The listing builds one solid part. Answer for the finished solid, in the listing's coordinates (mm). A direction names the side the tool comes from. Give positions to 0.01 mm unless a question says otherwise; leave off trailing zeros. Order: outer loops, then holes, each group sorted by start corner. A loop starts at its lowest first (then second) coordinate and runs counter-clockwise, first axis right, second up. Notation, with made-up numbers: (74.5, 83.5) -> (104.5, 83.5) arc R15 ccw to (104.5, 98.5) -> close; hole circle Ø7 at (18.5, 49.25). An arc over 180 degrees is marked (long way). One line per question, with ' | ' between items. Start each with the question number.
```python
from build123d import *

# Parameters (mm, degrees)
F1_DEPTH      = 208
F2_R          = 6
F3_DEPTH      = 65.001
F3_DEPTH_BACK = 5.001
F5_DEPTH      = 70
F6_R          = 6
F7_DEPTH      = 70.001
F8_R          = 4.05
F8_R_2        = 5
F9_DEPTH      = 40.001


with BuildPart() as f1:
    # F0 (on Front) → F1 (new body)
    with BuildSketch(Plane.XZ):
        with BuildLine():
            ThreePointArc((0, 30), (1.4644660941, 33.5355339059), (5, 35))
            Line((5, 35), (55, 35))
            ThreePointArc((55, 35), (58.5355339059, 33.5355339059), (60, 30))
            Line((60, 30), (60, 0))
            Line((60, 0), (65, 0))
            Line((65, 0), (65, 30))
            ThreePointArc((65, 30), (62.0710678119, 37.0710678119), (55, 40))
            Line((55, 40), (5, 40))
            ThreePointArc((5, 40), (-2.0710678119, 37.0710678119), (-5, 30))
            Line((-5, 30), (-5, 0))
            Line((-5, 0), (0, 0))
            Line((0, 0), (0, 30))
        make_face()
    extrude(amount=F1_DEPTH)

    # F2 (on Right) → F3 (cut, two sides)
    with BuildSketch(Plane.YZ) as f3_sk:
        with Locations((-196.0943733454, 12)):
            Circle(F2_R)
        with Locations((-156.0943733454, 12)):
            Circle(F2_R)
        with BuildLine():
            ThreePointArc((-34.0443733454, 12), (-38.0943733454, 16.05), (-42.1443733454, 12))
            ThreePointArc((-42.1443733454, 12), (-38.0943733454, 7.95), (-34.0443733454, 12))
        make_face()
        with BuildLine():
            ThreePointArc((-92.0443733454, 12), (-96.0943733454, 16.05), (-100.1443733454, 12))
            Line((-100.1443733454, 12), (-96.0943733454, 12))
            Line((-96.0943733454, 12), (-92.0443733454, 12))
        make_face()
        with BuildLine():
            Line((-96.0943733454, 12), (-100.1443733454, 12))
            ThreePointArc((-100.1443733454, 12), (-96.0943733454, 7.95), (-92.0443733454, 12))
            Line((-92.0443733454, 12), (-96.0943733454, 12))
        make_face()
    extrude(amount=F3_DEPTH, mode=Mode.SUBTRACT)
    extrude(f3_sk.sketch, amount=-F3_DEPTH_BACK, mode=Mode.SUBTRACT)

    # F4 (on Front) → F5 (join)
    with BuildSketch(Plane.XZ):
        Polygon((-5, 0), (0, 0), (0, 54), (0, 64), (-5, 64), (-5, 54), align=None)
        Polygon((60, 64), (60, 54), (60, 0), (65, 0), (65, 54), (65, 64), align=None)
    extrude(amount=-F5_DEPTH)

    # F6 (on face) → F7 (cut, through all)
    with BuildSketch(Plane(origin=(-5, 0, 0), x_dir=(0, -1, 0), z_dir=(-1, 0, 0))):
        with Locations((-60, 54)):
            Circle(F6_R)
        with Locations((-15.6066017178, 53.3933982822)):
            Circle(F6_R)
        with Locations((-60, 10)):
            Circle(F6_R)
        with Locations((-15.6066017178, 10.6066017178)):
            Circle(F6_R)
        with BuildLine():
            Line((-70, 10), (-70, 0))
            Line((-70, 0), (-60, 0))
            ThreePointArc((-60, 0), (-67.0710678119, 2.9289321881), (-70, 10))
        make_face()
        with BuildLine():
            ThreePointArc((208, 10), (205.0710678119, 2.9289321881), (198, 0))
            Line((198, 0), (208, 0))
            Line((208, 0), (208, 10))
        make_face()
        with BuildLine():
            Line((-70, 64), (-70, 54))
            ThreePointArc((-70, 54), (-67.0710678119, 61.0710678119), (-60, 64))
            Line((-60, 64), (-70, 64))
        make_face()
        with BuildLine():
            Line((-5, 64), (-15, 64))
            ThreePointArc((-15, 64), (-7.9289321881, 61.0710678119), (-5, 54))
            Line((-5, 54), (-5, 35))
            ThreePointArc((-5, 35), (-3.5355339059, 31.4644660941), (0, 30))
            Line((0, 30), (0, 63.4983927011))
            Line((0, 63.4983927011), (0, 64))
            Line((0, 64), (-5, 64))
        make_face()
    extrude(amount=-F7_DEPTH, mode=Mode.SUBTRACT)

    # F8 (on face) → F9 (cut, through all)
    with BuildSketch(Plane.XY.offset(40)):
        with Locations((15, -7)):
            Circle(F8_R)
        with Locations((15, -39)):
            Circle(F8_R)
        with Locations((15, -97)):
            Circle(F8_R)
        with BuildLine():
            Line((24.95, -76.95), (24.95, -97))
            Line((24.95, -97), (24.95, -117.05))
            ThreePointArc((24.95, -117.05), (30, -122.1), (35.05, -117.05))
            Line((35.05, -117.05), (35.05, -76.95))
            ThreePointArc((35.05, -76.95), (30, -71.9), (24.95, -76.95))
        make_face()
        with Locations((15, -155)):
            Circle(F8_R)
        with Locations((15, -200)):
            Circle(F8_R)
        with Locations((30, -200)):
            Circle(F8_R_2)
        with BuildLine():
            Line((35.05, -59.05), (35.05, -18.95))
            ThreePointArc((35.05, -18.95), (30, -13.9), (24.95, -18.95))
            Line((24.95, -18.95), (24.95, -59.05))
            ThreePointArc((24.95, -59.05), (30, -64.1), (35.05, -59.05))
        make_face()
        with BuildLine():
            ThreePointArc((24.95, -175.05), (30, -180.1), (35.05, -175.05))
            Line((35.05, -175.05), (35.05, -134.95))
            ThreePointArc((35.05, -134.95), (30, -129.9), (24.95, -134.95))
            Line((24.95, -134.95), (24.95, -175.05))
        make_face()
        with Locations((45, -7)):
            Circle(F8_R)
        with Locations((45, -39)):
            Circle(F8_R)
        with Locations((45, -97)):
            Circle(F8_R)
        with Locations((45, -155)):
            Circle(F8_R)
        with Locations((45, -200)):
            Circle(F8_R)
    extrude(amount=-F9_DEPTH, mode=Mode.SUBTRACT)


solid = f1.part
```
(1) Determine the mould class of faces 4 (the face through (35.05, -39, 38)), 5 (the face through (62.465, 16.907, 47.536)), 6 (the face through (-5, -40, 25)) for opening direction X: pulls with the +X half, pulls with the -X half, needs draft (parallel to the pull), parting line crosses it, or undercut.
(2) For faces 1 (the face through (-2.54, 8.01, 61.15)), 2 (the face through (29.9, -64.1, 37.5)), 3 (the face through (1, -103, 33)), determine the directions among +Z, -Z, +X, -X, +Y, -Y from which every point of the face is accessible in a straight line to the end or side of a thin tool.
(3) The part is cut by section B-B on z = 26. Determine the outline of the cut face in (x, y).
(4) Consider line 1 (X direction, y = -142, z = 15); line 2 (Z direction, x = -2.5, y = 60); line 3 (Z direction, x = 49.5, y = -166.5). Determine where each line is inside the solid, lowest interval first.
(5) The part is cut by section C-C on x = 14. Determine the outline of the cut face in (y, z), plus the area to 3 significant figures.
(6) Given P1, Ø1.5, axis at y = -94.5, z = 35, coming from the -X side; P2, Ø13, axis at x = 15, y = -97, coming from the +Z side; P3, Ø5.5, axis at x = -3.5, z = 45.5, coming from the -Y side; P4, Ø6.5, axis at y = -96.09, z = 12, coming from the +X side, each flat-ended and moving along its own axis, determine where each tip first touches the part or whether it passes through.
(7) The part is cut by section A-A on y = -7. Determine the outline of the cut face in (x, z).
(8) The part is cut by section D-D on x = 28.5. Determine the outline of the cut face in (y, z), plus the area to 3 significant figures.
Result sheet:
1) face 4: undercut | face 5: needs draft | face 6: pulls with the -X half
2) face 1: +Z, +X, -X, -Y | face 2: +Z, -Z | face 3: -Z, +Y, -Y
3) outline: (-5, -208) -> (0, -208) -> (0, 70) -> (-5, 70) -> close; (60, -208) -> (65, -208) -> (65, 70) -> (60, 70) -> close
4) line 1: x = -5 to 0, 60 to 65 | line 2: z = 0 to 4, 16 to 48, 60 to 64 | line 3: z = 35 to 40
5) outline: (-208, 35) -> (-203.92, 35) -> (-203.92, 40) -> (-208, 40) -> close; (-196.08, 35) -> (-158.92, 35) -> (-158.92, 40) -> (-196.08, 40) -> close; (-151.08, 35) -> (-100.92, 35) -> (-100.92, 40) -> (-151.08, 40) -> close; (-93.08, 35) -> (-42.92, 35) -> (-42.92, 40) -> (-93.08, 40) -> close; (-35.08, 35) -> (-10.92, 35) -> (-10.92, 40) -> (-35.08, 40) -> close; (-3.08, 35) -> (0, 35) -> (0, 40) -> (-3.08, 40) -> close | area: 844 mm^2
6) P1: stops at x = -4.05 | P2: stops at z = 40 | P3: stops at y = 5 | P4: passes through
7) outline: (-5, 0) -> (0, 0) -> (0, 30) arc R5 cw to (5, 35) -> (10.95, 35) -> (10.95, 40) -> (5, 40) arc R10 ccw to (-5, 30) -> close; (19.05, 35) -> (40.95, 35) -> (40.95, 40) -> (19.05, 40) -> close; (49.05, 35) -> (55, 35) arc R5 cw to (60, 30) -> (60, 0) -> (65, 0) -> (65, 30) arc R10 ccw to (55, 40) -> (49.05, 40) -> close
8) outline: (-208, 35) -> (-204.77, 35) -> (-204.77, 40) -> (-208, 40) -> close; (-195.23, 35) -> (-179.87, 35) -> (-179.87, 40) -> (-195.23, 40) -> close; (-130.13, 35) -> (-121.87, 35) -> (-121.87, 40) -> (-130.13, 40) -> close; (-72.13, 35) -> (-63.87, 35) -> (-63.87, 40) -> (-72.13, 40) -> close; (-14.13, 35) -> (0, 35) -> (0, 40) -> (-14.13, 40) -> close | area: 246 mm^2
